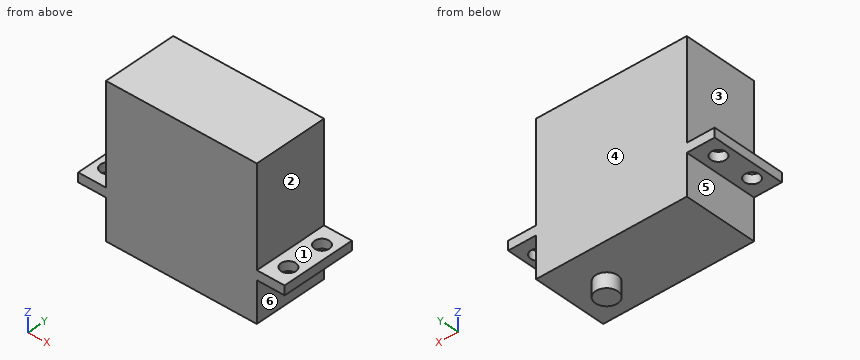
from build123d import *

# Parameters (mm, degrees)
SCHIZZO1_W                   = 40.7
SCHIZZO1_H                   = 20
ESTRUSIONE_ESTRUSIONE1_DEPTH = 40.3
SCHIZZO2_W                   = 2.5
SCHIZZO2_H                   = 20
ESTRUSIONE_ESTRUSIONE2_DEPTH = 7.5
RIPETIZIONE_A_L1_COUNT       = 2
RIPETIZIONE_A_L1_PITCH       = 48.2
SCHIZZO3_R                   = 3
ESTRUSIONE_ESTRUSIONE3_DEPTH = 4
SCHIZZO4_R                   = 2
TAGLIO_ESTRUSIONE1_DEPTH     = 10


with BuildPart() as part:
    # Schizzo1 → Estrusione-Estrusione1 (new body)
    with BuildSketch(Plane.XY):
        Rectangle(SCHIZZO1_W, SCHIZZO1_H)
    extrude(amount=ESTRUSIONE_ESTRUSIONE1_DEPTH)

    # Schizzo2 → Estrusione-Estrusione2 (add)
    with BuildSketch(Plane(origin=(20.35, 0, 0), x_dir=(0, 0, -1), z_dir=(1, 0, 0))):
        with Locations((-12.25, 0)):
            Rectangle(SCHIZZO2_W, SCHIZZO2_H)
    estrusione_estrusione2 = extrude(amount=ESTRUSIONE_ESTRUSIONE2_DEPTH)

    # Ripetizione a L1: Estrusione-Estrusione2 ×2
    with Locations(*[(-i * RIPETIZIONE_A_L1_PITCH, 0, 0) for i in range(1, RIPETIZIONE_A_L1_COUNT)]):
        add(estrusione_estrusione2)

    # Schizzo3 → Estrusione-Estrusione3 (add)
    with BuildSketch(Plane(origin=(0, 0, 0), x_dir=(-1, 0, 0), z_dir=(0, 0, -1))):
        with Locations((-10.35, 0)):
            Circle(SCHIZZO3_R)
    extrude(amount=ESTRUSIONE_ESTRUSIONE3_DEPTH)

    # Schizzo4 → Taglio-Estrusione1 (cut)
    with BuildSketch(Plane(origin=(0, 0, 11), x_dir=(-1, 0, 0), z_dir=(0, 0, -1))):
        with Locations((-24.35, 5)):
            Circle(SCHIZZO4_R)
        with Locations((-24.35, -5)):
            Circle(SCHIZZO4_R)
        with Locations((24.35, 5)):
            Circle(SCHIZZO4_R)
        with Locations((24.35, -5)):
            Circle(SCHIZZO4_R)
    extrude(amount=-TAGLIO_ESTRUSIONE1_DEPTH, mode=Mode.SUBTRACT)


solid = part.part
Verification items for the finished model (mm, model axes). Face numbers are marked on the shaded views. A direction names the side the tool comes from. Give positions to 0.01 mm unless a question says otherwise; leave off trailing zeros. Write each loop counter-clockwise with the first axis right and the second up, starting at its lowest first coordinate (ties: lowest second). Pieces come first, ordered by that corner, then holes.
(1) Mould release check, pull along X, two halves, no side actions. Record for the marked faces 1, 2 and 3: +X half, -X half, draft (parallel to the pull), parting line (faces both ways), or undercut.
(2) Gauge pin test, flat ends, axial feed: pin 1 (6.5 mm diameter, centred on x = -24.35, y = -5, fed in from +Z); pin 2 (8 mm diameter, centred on x = 24, y = -4, fed in from -Z); pin 3 (6.5 mm diameter, centred on x = 24.35, y = -5, fed in from -Z). Record the tip position at first contact, or that the pin passes through.
(3) Cross-section at C-C (x = -24.35). Enter the section's corners in (y, z), plus the area to 3 significant figures.
(4) Cross-section at A-A (y = 5). Enter the section's corners in (x, z).
(5) Cross-section at B-B (z = 12). Enter the section's corners in (x, y), plus the area to 3 significant figures.
(6) Cross-section at D-D (x = 10.35). Enter the section's corners in (y, z), plus the area to 3 significant figures.
(7) Material ranges on line 1 (Y direction, x = 24.35, z = 12.6); line 2 (X direction, y = 3.75, z = 12); line 3 (Z direction, x = -21, y = -3.25), recorded low to high.
(8) Access from +Z, -Z, +X, -X, +Y, -Y to the whole of each face (thin tool, end or side, straight path). Record for the marked faces 4, 5 and 6.
Worked out:
1. face 1: draft
1. face 2: +X half
1. face 3: -X half
2. pin 1: stops at z = 13.5
2. pin 2: stops at z = 0
2. pin 3: stops at z = 11
3. outline: (-10, 11) - (-7, 11) - (-7, 13.5) - (-10, 13.5) - close; (-3, 11) - (3, 11) - (3, 13.5) - (-3, 13.5) - close; (7, 11) - (10, 11) - (10, 13.5) - (7, 13.5) - close
3. area: 30.0 mm2
4. outline: (-27.85, 11) - (-26.35, 11) - (-26.35, 13.5) - (-27.85, 13.5) - close; (-22.35, 11) - (-20.35, 11) - (-20.35, 0) - (20.35, 0) - (20.35, 11) - (22.35, 11) - (22.35, 13.5) - (20.35, 13.5) - (20.35, 40.3) - (-20.35, 40.3) - (-20.35, 13.5) - (-22.35, 13.5) - close; (26.35, 11) - (27.85, 11) - (27.85, 13.5) - (26.35, 13.5) - close
5. outline: (-27.85, -10) - (27.85, -10) - (27.85, 10) - (-27.85, 10) - close; hole circle Ø4 at (-24.35, -5); hole circle Ø4 at (-24.35, 5); hole circle Ø4 at (24.35, -5); hole circle Ø4 at (24.35, 5)
5. area: 1,060 mm2
6. outline: (-10, 0) - (-3, 0) - (-3, -4) - (3, -4) - (3, 0) - (10, 0) - (10, 40.3) - (-10, 40.3) - close
6. area: 830 mm2
7. line 1: y = -10 to -7, -3 to 3, 7 to 10
7. line 2: x = -27.85 to -25.91, -22.79 to 22.79, 25.91 to 27.85
7. line 3: z = 11 to 13.5
8. face 4: +Z, -Z, +X, -X, +Y
8. face 5: -Z, -X, +Y, -Y
8. face 6: -Z, +X, +Y, -Y
